For this review, take the finished solid that the model builds, in its own axes (mm). Face numbers are marked on the shaded views. A direction names the side the tool comes from. Coordinates: 2 decimals unless noted, no trailing zeros. Loops run counter-clockwise (first coordinate to the right, second up) from the corner with the lowest first, then second, coordinate; pieces in that order, holes last. Notation, with made-up numbers: M 16.5,39.25 L 69.5,39.25 A30 cw 69.5,72.25 Z; hole C 27.25,43 d11. An arc over 180 degrees is marked long. Put each result on its own line as item: value.
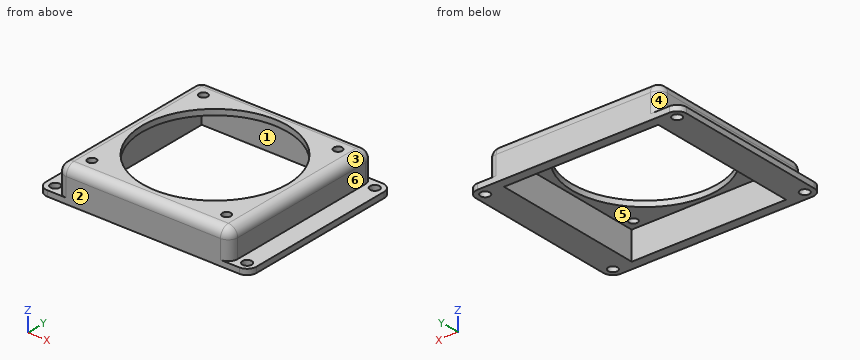
```python
from build123d import *

# Parameters (mm, degrees)
SKETCH1_W           = 92
SKETCH1_H           = 92
SKETCH1_R           = 38.7
SKETCH1_R_2         = 2.25
BOSS_EXTRUDE1_DEPTH = 3
SKETCH2_W           = 92
SKETCH2_H           = 92
SKETCH2_W_2         = 82
SKETCH2_H_2         = 82
BOSS_EXTRUDE2_DEPTH = 15
SKETCH3_W           = 10
SKETCH3_H           = 92
SKETCH3_R           = 2.5
BOSS_EXTRUDE3_DEPTH = 3
FILLET1_R           = 5


with BuildPart() as part:
    # Sketch1 → Boss-Extrude1 (new body)
    with BuildSketch(Plane.XY):
        Rectangle(SKETCH1_W, SKETCH1_H)
        Circle(SKETCH1_R, mode=Mode.SUBTRACT)
        with Locations((-35.78, 35.78)):
            Circle(SKETCH1_R_2, mode=Mode.SUBTRACT)
        with Locations((35.78, 35.78)):
            Circle(SKETCH1_R_2, mode=Mode.SUBTRACT)
        with Locations((35.78, -35.78)):
            Circle(SKETCH1_R_2, mode=Mode.SUBTRACT)
        with Locations((-35.78, -35.78)):
            Circle(SKETCH1_R_2, mode=Mode.SUBTRACT)
    extrude(amount=BOSS_EXTRUDE1_DEPTH)

    # Sketch2 → Boss-Extrude2 (add)
    with BuildSketch(Plane(origin=(0, 0, 0), x_dir=(-1, 0, 0), z_dir=(0, 0, -1))):
        Rectangle(SKETCH2_W, SKETCH2_H)
        Rectangle(SKETCH2_W_2, SKETCH2_H_2, mode=Mode.SUBTRACT)
    extrude(amount=BOSS_EXTRUDE2_DEPTH)

    # Sketch3 → Boss-Extrude3 (add)
    # profile 1 of 2: a face of its own
    with BuildSketch(Plane(origin=(0, 0, -15), x_dir=(-1, 0, 0), z_dir=(0, 0, -1))):
        with Locations((-51, 0)):
            Rectangle(SKETCH3_W, SKETCH3_H)
        with Locations((-51, 41)):
            Circle(SKETCH3_R, mode=Mode.SUBTRACT)
        with Locations((-51, -41)):
            Circle(SKETCH3_R, mode=Mode.SUBTRACT)
    # profile 2 of 2: a face of its own
    with BuildSketch(Plane(origin=(0, 0, -15), x_dir=(-1, 0, 0), z_dir=(0, 0, -1))):
        with Locations((51, 0)):
            Rectangle(SKETCH3_W, SKETCH3_H)
        with Locations((51, 41)):
            Circle(SKETCH3_R, mode=Mode.SUBTRACT)
        with Locations((51, -41)):
            Circle(SKETCH3_R, mode=Mode.SUBTRACT)
    extrude(amount=-BOSS_EXTRUDE3_DEPTH)

    # Fillet1
    fillet1_edges = [part.edges().sort_by_distance(p)[0] for p in [
        (46, 0, 3),
        (0, 46, 3),
        (-46, 0, 3),
        (56, -46, -13.5),
        (56, 46, -13.5),
        (-56, 46, -13.5),
        (-56, -46, -13.5),
        (-46, 46, -4.5),
        (46, 46, -4.5),
        (46, -46, -4.5),
        (-46, -46, -4.5),
        (0, -46, 3),
    ]]
    fillet(fillet1_edges, radius=FILLET1_R)


solid = part.part
```
(1) Tool access review of the marked faces 4, 5 and 6: name each direction out of +Z, -Z, +X, -X, +Y, -Y from which nothing blocks a thin tool from reaching the whole face with its end or side.
Determined:
face 4: +Z, -X, +Y
face 5: -Z
face 6: +Z, +X, +Y, -Y
(2) Add section B-B (y = -23.5). Write out the cut boundary in (x, z), plus the area to 3 significant figures.
Determined:
outline: M -56,-15 L -41,-15 L -41,0 L -30.75,0 L -30.75,3 L -41,3 A5 ccw -46,-2 L -46,-12 L -56,-12 Z; M 30.75,0 L 41,0 L 41,-15 L 56,-15 L 56,-12 L 46,-12 L 46,-2 A5 ccw 41,3 L 30.75,3 Z
area: 291 mm^2
(3) Add section D-D (x = -44). Write out the cut boundary in (y, z), plus the area to 3 significant figures.
Determined:
outline: M -46,-15 L 46,-15 L 46,-12 L 45,-12 L 45,-2 A4 ccw 41,2 L -41,2 A4 ccw -45,-2 L -45,-12 L -46,-12 Z
area: 1,530 mm^2
(4) Wall thickness on line 1 along Y through (x, z) = (51, -13.1); line 2 along X through (y, z) = (-17, -11.25): over which ranges is each line inside the solid? List them lowest first. Write a range as [from, to].
Determined:
line 1: y = [-46, -43.5], [-38.5, 38.5], [43.5, 46]
line 2: x = [-46, -41], [41, 46]
(5) Add section A-A (x = -19). Write out the cut boundary in (y, z).
Determined:
outline: M -46,-15 L -41,-15 L -41,0 L -33.71,0 L -33.71,3 L -41,3 A5 ccw -46,-2 Z; M 33.71,0 L 41,0 L 41,-15 L 46,-15 L 46,-2 A5 ccw 41,3 L 33.71,3 Z
(6) Add section C-C (z = -3.5). Write out the cut boundary in (x, y).
Determined:
outline: M -46,-41 A5 ccw -41,-46 L 41,-46 A5 ccw 46,-41 L 46,41 A5 ccw 41,46 L -41,46 A5 ccw -46,41 Z; hole M -41,-41 L 41,-41 L 41,41 L -41,41 Z
(7) Draft analysis for pull direction Y (two halves, no side actions). For the marked faces 1, 2 and 3, state which applies: +Y half, -Y half, draft (parallel to the pull), parting line (faces both ways), or undercut.
Determined:
face 1: undercut
face 2: -Y half
face 3: draft
(8) For pin 1 (7 mm diameter, centred on x = -35.78, y = 35.78, fed in from -Z); pin 2 (6 mm diameter, centred on x = -51, y = 41, fed in from +Z); pin 3 (4.5 mm diameter, centred on x = -47.5, y = -17, fed in from +Z), all flat-tipped, find the tip position at first contact; note any pin that passes through.
Determined:
pin 1: stops at z = 0
pin 2: stops at z = -12
pin 3: stops at z = 0.63
